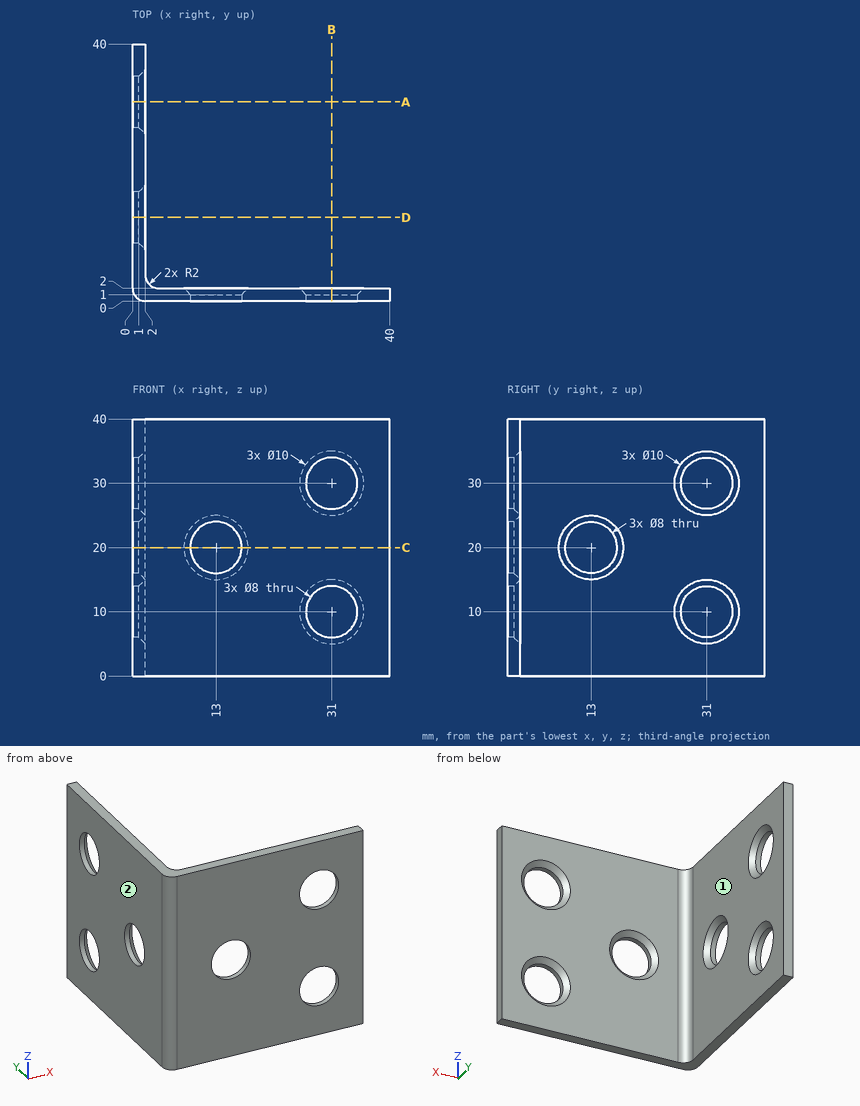
The drawing under review shows one solid part. Ordinate dimensions are in mm from its lowest x, y, z. A direction names the side the tool comes from. Round coordinates to 2 decimals unless told otherwise and drop trailing zeros. Loops run counter-clockwise (first coordinate to the right, second up) from the corner with the lowest first, then second, coordinate; pieces in that order, holes last. Notation, with made-up numbers: (55, 27.25) - (86, 27.25) arc R27 cw to (86, 58.25) - close; hole circle Ø11 at (-4, -40). An arc over 180 degrees is marked (long way). One line per item, written item: value. Start each with the question number.
1) Consider section A-A on y = 31. Give the boundary of the cut face in (x, z).
2) Insertion check: pin 1 Ø1.5 at (x, z) = (24, 24.5) entering from -Y; pin 2 Ø5 at (y, z) = (13, 20) entering from -X; pin 3 Ø11 at (y, z) = (18.5, 24.5) entering from +X; pin 4 Ø1 at (x, z) = (35.5, 34) entering from +Y. Each pin has a flat end and moves straight along its axis. Give the tip position at first contact, or say it passes through.
3) Consider section D-D on y = 13. Give the boundary of the cut face in (x, z), then the cut area to 3 significant figures.
4) To check wall thickness, follow L1, parallel to Z at x = 0.2, y = 31; L2, parallel to Z at x = 13, y = 0.45; L3, parallel to X at y = 11, z = 5.5. State the ranges of each line that lie inside material, in increasing order. Write a range as from..to.
5) Consider section C-C on z = 20. Give the boundary of the cut face in (x, y).
6) For the marked faces 1 and 2, list the 3-axis set-ups (+Z, -Z, +X, -X, +Y, -Y) from which the entire face can be reached by the end or side of a thin tool; tool diameter is ignored.
Reported:
1. outline: (0, 0) - (2, 0) - (2, 5) - (1, 6) - (0, 6) - close; (0, 14) - (1, 14) - (2, 15) - (2, 25) - (1, 26) - (0, 26) - close; (0, 34) - (1, 34) - (2, 35) - (2, 40) - (0, 40) - close
2. pin 1: stops at y = 0
2. pin 2: passes through
2. pin 3: stops at x = 2
2. pin 4: stops at y = 2
3. outline: (0, 0) - (2, 0) - (2, 15) - (1, 16) - (0, 16) - close; (0, 24) - (1, 24) - (2, 25) - (2, 40) - (0, 40) - close
3. area: 63.0 mm^2
4. L1: z = 0..6, 14..26, 34..40
4. L2: z = 0..16, 24..40
4. L3: x = 0..2
5. outline: (0, 2) arc R2 ccw to (2, 0) - (9, 0) - (9, 1) - (8, 2) - (4, 2) arc R2 cw to (2, 4) - (2, 8) - (1, 9) - (0, 9) - close; (0, 17) - (1, 17) - (2, 18) - (2, 40) - (0, 40) - close; (17, 0) - (40, 0) - (40, 2) - (18, 2) - (17, 1) - close
6. face 1: +Z, -Z, +X, +Y
6. face 2: +Z, -Z, -X, +Y, -Y
